Geometry check sheet. Reference: drawing and pictorial views, mm from the part's lowest x, y, z. A direction names the side the tool comes from. Round coordinates to 2 decimals unless told otherwise and drop trailing zeros. Write each loop counter-clockwise with the first axis right and the second up, starting at its lowest first coordinate (ties: lowest second). Pieces come first, ordered by that corner, then holes. Notation, with made-up numbers: M 59,78.5 L 111,78.5 A27 ccw 111,115.5 Z; hole C -16.5,26 d10. An arc over 180 degrees is marked long. Put each result on its own line as item: value. Start each with the question number.
(1) Tool access check on the marked faces 1 and 2. Record the directions out of +Z, -Z, +X, -X, +Y, -Y that give a thin tool (end or side, any length) a straight path to the whole face; none if there is none.
(2) Section check D-D on z = 10. Record the cut outline in (x, y).
(3) Gauge pin test, flat ends, axial feed: pin 1 (3 mm diameter, centred on y = 7.5, z = 27, fed in from +X); pin 2 (10 mm diameter, centred on x = 6, y = 36, fed in from +Z); pin 3 (10 mm diameter, centred on x = 14, z = 62.5, fed in from +Y). Record the tip position at first contact, or that the pin passes through.
(4) Section check B-B on z = 74.49. Record the cut outline in (x, y) (3 decimals), then the cut area to 3 significant figures.
(5) Material ranges on probe 1 along Z at (x, y) = (18, 1.8); probe 2 along Y at (x, z) = (1.3, 95.49) (1 decimal); probe 3 along X at (y, z) = (28, 53), recorded low to high.
(6) Section check C-C on x = 18. Record the cut outline in (y, z), then the cut area to 3 significant figures.
(7) Section check A-A on x = 24. Record the cut outline in (y, z).
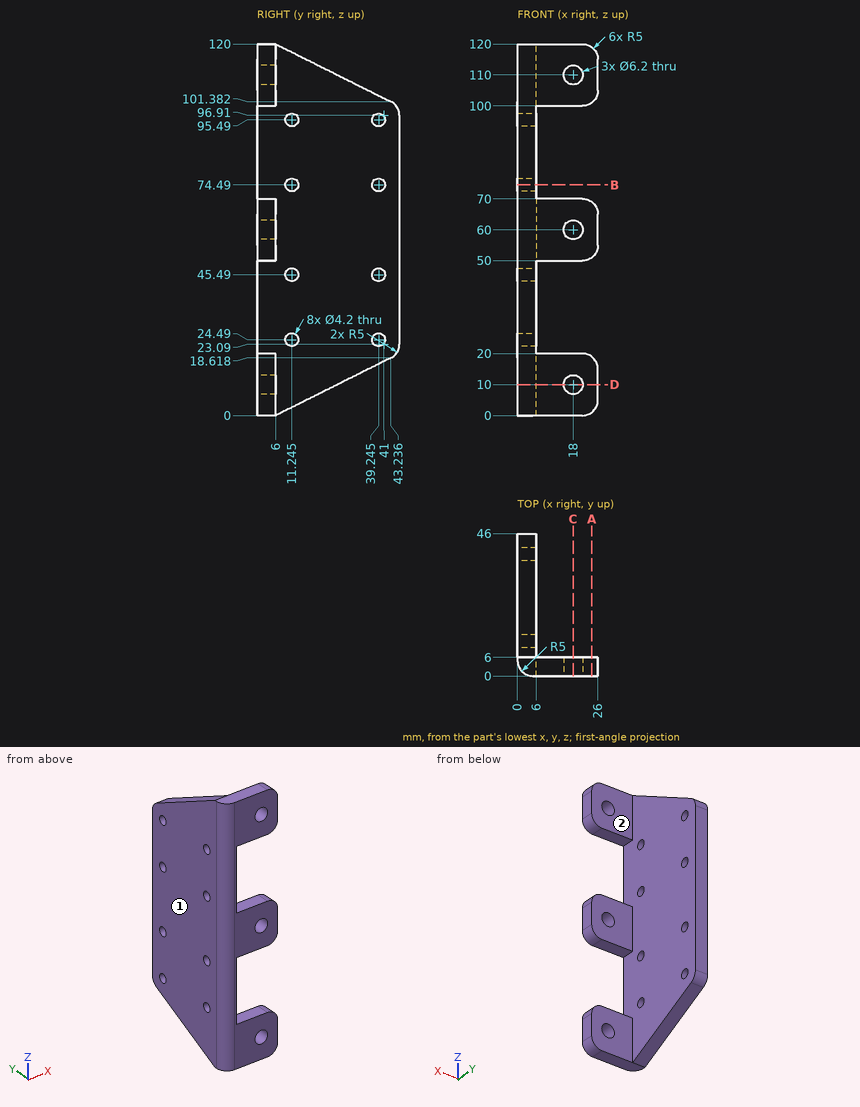
Answers follow:
1. face 1: +Z, -Z, -X, +Y, -Y
1. face 2: +Z, -Z, +X, +Y
2. outline: M 0,5 A5 ccw 5,0 L 14.9,0 L 14.9,6 L 6,6 L 6,26 L 0,26 Z; M 21.1,0 L 26,0 L 26,6 L 21.1,6 Z
3. pin 1: stops at x = 6
3. pin 2: stops at z = 107.5
3. pin 3: stops at y = 6
4. outline: M 0,5 A5 ccw 5,0 L 6,0 L 6,9.145 L 0,9.145 Z; M 0,13.345 L 6,13.345 L 6,37.145 L 0,37.145 Z; M 0,41.345 L 6,41.345 L 6,46 L 0,46 Z
4. area: 220 mm^2
5. probe 1: z = 0 to 6.9, 13.1 to 20, 50 to 56.9, 63.1 to 70, 100 to 106.9, 113.1 to 120
5. probe 2: y = 1.6 to 9.1, 13.3 to 37.1, 41.3 to 46
5. probe 3: x = 0 to 6
6. outline: M 0,0 L 6,0 L 6,6.9 L 0,6.9 Z; M 0,13.1 L 6,13.1 L 6,20 L 0,20 Z; M 0,50 L 6,50 L 6,56.9 L 0,56.9 Z; M 0,63.1 L 6,63.1 L 6,70 L 0,70 Z; M 0,100 L 6,100 L 6,106.9 L 0,106.9 Z; M 0,113.1 L 6,113.1 L 6,120 L 0,120 Z
6. area: 248 mm^2
7. outline: M 0,1 L 6,1 L 6,19 L 0,19 Z; M 0,51 L 6,51 L 6,69 L 0,69 Z; M 0,101 L 6,101 L 6,119 L 0,119 Z
